Design review of the part built by this model. Coordinates are the model's own, in mm. Face numbers are marked on the shaded views. A direction names the side the tool comes from. Round coordinates to 2 decimals unless told otherwise and drop trailing zeros. Loops run counter-clockwise (first coordinate to the right, second up) from the corner with the lowest first, then second, coordinate; pieces in that order, holes last. Notation, with made-up numbers: (19, -32.5) -> (48, -32.5) arc R24 cw to (48, -8.5) -> close; hole circle Ø2 at (76.5, 53.5). An arc over 180 degrees is marked (long way). Answer as CSV lines item,"result". Start each with the question number.
(1) To check wall thickness, follow line 1 (Y direction, x = 7.25, z = 2.35) (3 decimals); line 2 (X direction, y = -2.25, z = 2.15) (3 decimals). State the ranges of each line that lie inside material, in increasing order. Write a range as from..to.
(2) For P1, Ø1.6, axis at x = 0, y = -0.5, coming from the +Z side, flat-tipped, find the tip position at first contact; note if it passes through.
(3) Take a section at A-A, the plane z = 3.1. Write out the cut boundary in (x, y) (3 decimals).
(4) Take a section at D-D, the plane z = 1.75. Write out the cut boundary in (x, y) (3 decimals), and give its area (3 significant figures).
(5) Machinability: for the marked faces 4 and 5, which of the approach directions +Z, -Z, +X, -X, +Y, -Y give a long, thin tool a straight path to every point of the face, cutting with its end or side? Answer none if there is none.
(6) Take a section at B-B, the plane y = -0.5. Write out the cut boundary in (x, z) (3 decimals).
(7) Draft analysis for pull direction X (two halves, no side actions). For the marked faces 1, 2 and 3, state which applies: +X half, -X half, draft (parallel to the pull), parting line (faces both ways), or undercut.
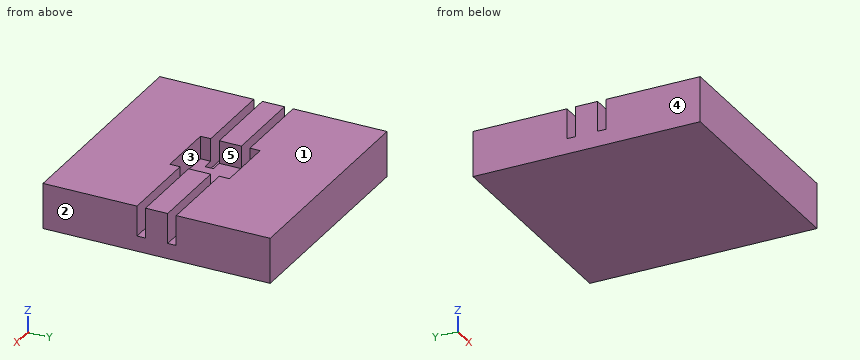
from build123d import *

# Parameters (mm, degrees)
F0_W     = 20
F0_H     = 20
F1_DEPTH = 4
F2_W     = 5.25
F2_H     = 5.25
F3_DEPTH = 2
F4_W     = 8.375
F4_H     = 0.75
F5_DEPTH = 2.65


with BuildPart() as f1:
    # F0 (on Top) → F1 (new body)
    with BuildSketch(Plane.XY):
        Rectangle(F0_W, F0_H)
    extrude(amount=F1_DEPTH)

    # F2 (on face) → F3 (cut)
    with BuildSketch(Plane.XY.offset(4)):
        Rectangle(F2_W, F2_H)
    extrude(amount=-F3_DEPTH, mode=Mode.SUBTRACT)

    # F4 (on face) → F5 (cut)
    with BuildSketch(Plane.XY.offset(4)):
        with Locations((-5.8125, 1.35)):
            Rectangle(F4_W, F4_H)
        with Locations((5.8125, 1.35)):
            Rectangle(F4_W, F4_H)
        with Locations((5.8125, -1.35)):
            Rectangle(F4_W, F4_H)
        with Locations((-5.8125, -1.35)):
            Rectangle(F4_W, F4_H)
    extrude(amount=-F5_DEPTH, mode=Mode.SUBTRACT)


solid = f1.part
The answers:
1,line 1,"-10..-1.725, -0.975..0.975, 1.725..10"
1,line 2,"-10..-2.625, 2.625..10"
2,P1,"z = 2"
3,outline,"(-10, -10) -> (10, -10) -> (10, -1.725) -> (2.625, -1.725) -> (2.625, -2.625) -> (-2.625, -2.625) -> (-2.625, -1.725) -> (-10, -1.725) -> close; (-10, -0.975) -> (-2.625, -0.975) -> (-2.625, 0.975) -> (-10, 0.975) -> close; (-10, 1.725) -> (-2.625, 1.725) -> (-2.625, 2.625) -> (2.625, 2.625) -> (2.625, 1.725) -> (10, 1.725) -> (10, 10) -> (-10, 10) -> close; (2.625, -0.975) -> (10, -0.975) -> (10, 0.975) -> (2.625, 0.975) -> close"
4,outline,"(-10, -10) -> (10, -10) -> (10, -1.725) -> (1.625, -1.725) -> (1.625, -0.975) -> (10, -0.975) -> (10, 0.975) -> (1.625, 0.975) -> (1.625, 1.725) -> (10, 1.725) -> (10, 10) -> (-10, 10) -> (-10, 1.725) -> (-1.625, 1.725) -> (-1.625, 0.975) -> (-10, 0.975) -> (-10, -0.975) -> (-1.625, -0.975) -> (-1.625, -1.725) -> (-10, -1.725) -> close"
4,area,"375 mm²"
5,face 4,"+Z, -Z, -X, +Y, -Y"
5,face 5,"+Z"
6,outline,"(-10, 0) -> (10, 0) -> (10, 4) -> (2.625, 4) -> (2.625, 2) -> (-2.625, 2) -> (-2.625, 4) -> (-10, 4) -> close"
7,face 1,"draft"
7,face 2,"+X half"
7,face 3,"undercut"
